CAD build for the part. Positions are in the model's coordinates, mm. A direction names the side the tool comes from. Coordinates: 2 decimals unless noted, no trailing zeros. Loops run counter-clockwise (first coordinate to the right, second up) from the corner with the lowest first, then second, coordinate; pieces in that order, holes last.
1) Saw through at B-B, the plane z = 0. Write the cut outline in (x, y), and give its area (3 significant figures).
2) Saw through at C-C, the plane x = 45. Write the cut outline in (y, z), and give its area (3 significant figures).
3) Saw through at A-A, the plane y = 0. Write the cut outline in (x, z).
4) Which spindle directions (+Z, -Z, +X, -X, +Y, -Y) get a long thin tool onto all of the face, cutting with end or side? Do faces 1 (the cylindrical face through (23.731, -1.802, -5.723)), 2 (the cylindrical face through (48.1, 1.72, -4.16)), 3 (the cylindrical face through (4.03, -3.04, 3.32)). Say none if no direction does.
5) Two-plate mould, pull along X, no slides. Class faces 4 (the flat face through (0, 0, 0)), 5 (the cylindrical face through (50.464, 0.325, -0.062)), 6 (the flat face through (56, 0, 0)): +X half, -X half, draft (parallel to the pull), parting line (faces both ways), or undercut.
6) Pin check, flat tips, straight feed: pin 1 Ø2 at (x, z) = (37.5, 0.5) entering from +Y; pin 2 Ø2 at (x, z) = (34, -3.5) entering from +Y; pin 3 Ø4 at (x, y) = (49, 0) entering from +Z; pin 4 Ø4 at (x, z) = (16.5, -4) entering from -Y. Stop position of each tip, or through.
7) Saw through at D-D, the plane x = 8. Write the cut outline in (y, z).
8) Wall check: line 1 along X through (y, z) = (0, -0.25); line 2 along X through (y, z) = (1.25, -4.5); line 3 along Y through (x, z) = (49, -1.5). Give the ranges that are in metal, low to high.
```python
from build123d import *

# Parameters (mm, degrees)
CHAMFER2_SIZE            = 1
FILLET1_R                = 2
F_3_0_3_DIAMETER_HOLE1_D = 3


with BuildPart() as part:
    # Sketch1 → Revolve1 (revolve)
    with BuildSketch(Plane.XY, mode=Mode.PRIVATE) as revolve1_sk:
        Polygon((0, 0), (0, 4.5), (6, 4.5), (6, 6), (41, 6), (41, 4.5), (56, 4.5), (56, 0), align=None)
    revolve(revolve1_sk.sketch.rotate(Axis((0, 0, 0), (-1, 0, 0)), 90), axis=Axis((0, 0, 0), (-1, 0, 0)))

    # Chamfer2
    chamfer2_edges = [part.edges().sort_by_distance(p)[0] for p in [
        (56, 0, 4.5),
        (41, 0, 6),
        (6, 0, 6),
    ]]
    chamfer(chamfer2_edges, length=CHAMFER2_SIZE)

    # Fillet1
    fillet1_edges = [part.edges().sort_by_distance(p)[0] for p in [
        (0, 0, 4.5),
    ]]
    fillet(fillet1_edges, radius=FILLET1_R)

    # Ø3.0 (3) Diameter Hole1 (through all)
    with Locations(Plane(origin=(49, 0, 4.5), x_dir=(0, 1, 0), z_dir=(0, 0, 1))):
        with Locations((0, 0)):
            Hole(F_3_0_3_DIAMETER_HOLE1_D / 2)


solid = part.part
```
Data:
1. outline: (0, -2.5) arc R2 ccw to (2, -4.5) - (6, -4.5) - (6, -5) - (7, -6) - (40, -6) - (41, -5) - (41, -4.5) - (55, -4.5) - (56, -3.5) - (56, 3.5) - (55, 4.5) - (41, 4.5) - (41, 5) - (40, 6) - (7, 6) - (6, 5) - (6, 4.5) - (2, 4.5) arc R2 ccw to (0, 2.5) - close; hole circle Ø3 at (49, 0)
1. area: 597 mm2
2. outline: circle Ø9 at (0, 0)
2. area: 63.6 mm2
3. outline: (0, -2.5) arc R2 ccw to (2, -4.5) - (6, -4.5) - (6, -5) - (7, -6) - (40, -6) - (41, -5) - (41, -4.5) - (47.5, -4.5) - (47.5, 4.5) - (41, 4.5) - (41, 5) - (40, 6) - (7, 6) - (6, 5) - (6, 4.5) - (2, 4.5) arc R2 ccw to (0, 2.5) - close; (50.5, -4.5) - (55, -4.5) - (56, -3.5) - (56, 3.5) - (55, 4.5) - (50.5, 4.5) - close
4. face 1: +X, -X
4. face 2: +X
4. face 3: -X
5. face 4: -X half
5. face 5: undercut
5. face 6: +X half
6. pin 1: stops at y = 6
6. pin 2: stops at y = 5.45
6. pin 3: stops at z = 4.5
6. pin 4: stops at y = -5.66
7. outline: circle Ø12 at (0, 0)
8. line 1: x = 0 to 47.5, 50.5 to 56
8. line 2: x = 6 to 41
8. line 3: y = -4.24 to -1.5, 1.5 to 4.24
